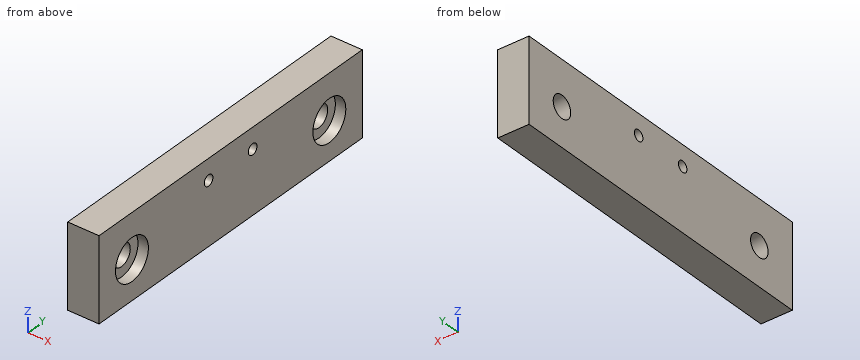
Autodesk Inventor part; units mm, degrees
ref_plane "YZ Plane" through (0, 0, 0) normal (1, 0, 0) x (0, 1, 0)
ref_plane "XZ Plane" through (0, 0, 0) normal (0, 1, 0) x (-1, 0, 0)
ref_plane "XY Plane" through (0, 0, 0) normal (0, 0, 1) x (1, 0, 0)
sketch "Sketch1" plane through (0, 0, 0) normal (1, 0, 0) x (0, 1, 0)
  line L0 (0, 0) -> (101.6, 0)
  line L1 (101.6, 0) -> (101.6, -25.4)
  line L2 (101.6, -25.4) -> (0, -25.4)
  line L3 (0, -25.4) -> (0, 0)
  point P0 (95.25, -12.7)
  point P1 (6.35, -12.7)
  dimension "d0" = 25.4
  dimension "d1" = 101.6
  dimension "d4" = 6.35
  dimension "d5" = 12.7
  dimension "d6" = 6.35
extrude "Extrusion1" add sketch "Sketch1" along normal blind 9.525
sketch "Sketch2" plane through (9.525, 0, 0) normal (1, 0, 0) x (0, 0, -1)
  line L0 (25.4, 101.6) -> (0, 101.6)
  point P0 (0, 0)
  point P1 (13.6787, 88.9)
  dimension "d22" = 12.7
hole "Hole1" at (9.525, 88.9, -13.6787) direction (-1, 0, 0) diameter 6.7564 end through all counterbore diameter 12.7 counterbore depth 3.175
sketch "Sketch3" plane through (9.525, 0, 0) normal (1, 0, 0) x (0, 0, -1)
  line L0 (0, 0) -> (25.4, 0)
  point P0 (13.5273, 12.7)
  dimension "d21" = 12.7
hole "Hole2" at (9.525, 12.7, -13.5273) direction (-1, 0, 0) diameter 6.7564 end through all counterbore diameter 12.7 counterbore depth 3.175
sketch "Sketch4" plane through (9.525, 0, 0) normal (1, 0, 0) x (0, 0, -1)
  line L0 (0, 101.6) -> (0, 0)
  line L1 (25.4, 101.6) -> (0, 101.6)
  point P0 (6.35, 59.3)
  dimension "d30" = 6.35
  dimension "d31" = 42.3
hole "Hole3" at (9.525, 59.3, -6.35) direction (-1, 0, 0) diameter 3.302 end through all
sketch "Sketch5" plane through (9.525, 0, 0) normal (1, 0, 0) x (0, 0, -1)
  line L0 (0, 0) -> (25.4, 0)
  line L1 (0, 101.6) -> (0, 0)
  point P0 (6.35, 42.3)
  dimension "d39" = 42.3
  dimension "d40" = 6.35
hole "Hole4" at (9.525, 42.3, -6.35) direction (-1, 0, 0) diameter 3.302 end through all
properties part number "NeedleValvePanel V1"
Here's how the part is built. I have some questions about the finished solid (model axes, mm). Coordinates: 2 decimals unless noted, no trailing zeros. Write each loop counter-clockwise with the first axis right and the second up, starting at its lowest first coordinate (ties: lowest second). Pieces come first, ordered by that corner, then holes.
Item 1: I want a section at A-A on y = 59.3. Write out the boundary of the cut face in (x, z) (3 decimals).
Item 2: I want a section at B-B on x = 7.5. Write out the boundary of the cut face in (y, z), and give its area (3 significant figures).
Item 3: Will this pin go through, and if not, where does the flat tip stop? pin 1 (7.5 mm diameter, centred on y = 88.9, z = -13.68, fed in from +X).
Item 4: I want a section at C-C on z = -13.5. Write out the boundary of the cut face in (x, y) (3 decimals).
Item 5: If I drill on line 1 (Y direction, x = 3.25, z = -6.5); line 2 (Y direction, x = 7, z = -6.35); line 3 (Z direction, x = 3.75, y = 12.7), over which ranges is the centre line in solid material (lowest first)?
Findings below:
1. outline: (0, -25.4) - (9.525, -25.4) - (9.525, -8.001) - (0, -8.001) - close; (0, -4.699) - (9.525, -4.699) - (9.525, 0) - (0, 0) - close
2. outline: (0, -25.4) - (101.6, -25.4) - (101.6, 0) - (0, 0) - close; hole circle Ø12.7 at (12.7, -13.53); hole circle Ø3.3 at (42.3, -6.35); hole circle Ø3.3 at (59.3, -6.35); hole circle Ø12.7 at (88.9, -13.68)
2. area: 2,310 mm2
3. pin 1: stops at x = 6.35
4. outline: (0, 0) - (9.525, 0) - (9.525, 6.35) - (6.35, 6.35) - (6.35, 9.322) - (0, 9.322) - close; (0, 16.078) - (6.35, 16.078) - (6.35, 19.05) - (9.525, 19.05) - (9.525, 82.553) - (6.35, 82.553) - (6.35, 85.527) - (0, 85.527) - close; (0, 92.273) - (6.35, 92.273) - (6.35, 95.247) - (9.525, 95.247) - (9.525, 101.6) - (0, 101.6) - close
5. line 1: y = 0 to 40.66, 43.94 to 57.66, 60.94 to 101.6
5. line 2: y = 0 to 40.65, 43.95 to 57.65, 60.95 to 101.6
5. line 3: z = -25.4 to -16.91, -10.15 to 0
